Autodesk Fusion 360 part; units mm, degrees
sketch "Sketch1" plane through (0, 0, 0) normal (0, 0, 1) x (1, 0, 0)
  circle A0 centre (0, 0) radius 31.75
  circle A1 centre (0, 0) radius 25.4
  dimension "d1" = 63.5
  dimension "d2" = 50.8
extrude "Extrude1" add sketch "Sketch1" along normal blind 7.62 makes body 1
chamfer "Chamfer1" distance 3.175 distance2 3.175 1 edges at (-23.6811, 9.185, 7.62) measured on face at (29.4206, -2.8393, 7.62) on bodies 1
sketch "Sketch2" plane through (0, 0, 0) normal (1, 0, 0) x (0, 1, 0)
  arc A0 (-31.115, 59.4476) -> (-33.147, 7.7483) centre (-9.0465, 32.6906) ccw
  arc A1 (-46.5417, 59.4476) -> (-33.147, 0) centre (-13.9818, 35.5511) ccw
  line L0 (-33.147, 7.7483) -> (-33.147, 0)
  line L1 (-33.147, 7.7483) -> (-29.083, 7.7483)
  line L2 (-29.083, 7.7483) -> (-29.083, 0)
  line L3 (-29.083, 0) -> (-33.147, 0)
  line L4 (-33.147, 0) -> (-33.147, 7.7483)
  line L5 (-31.115, 0) -> (-31.115, 59.4476) construction
  line L6 (-46.5417, 59.4476) -> (-31.115, 59.4476)
extrude "Extrude2" add sketch "Sketch2" along normal blind 7.62 bodies 1
sketch "Sketch5" plane through (0, 0, 59.4476) normal (0, 0, 1) x (-1, 0, 0)
  line L0 (0, 31.115) -> (0, 46.5417)
  line L1 (0, 46.5417) -> (-7.62, 46.5417)
  line L2 (-7.62, 46.5417) -> (-7.62, 31.115)
  line L3 (-7.62, 31.115) -> (0, 31.115)
  line L4 (12.7, 39.2684) -> (-12.7, 39.2684) construction
  line L5 (-12.7, 39.2684) -> (-12.7, -39.2684) construction
  line L6 (-12.7, -39.2684) -> (12.7, -39.2684) construction
  line L7 (12.7, -39.2684) -> (12.7, 39.2684) construction
  line L8 (12.7, 39.2684) -> (-12.7, -39.2684) construction
  line L9 (-12.7, 39.2684) -> (12.7, -39.2684) construction
  arc A0 (12.7, -39.2684) -> (12.7, 39.2684) centre (-69.8788, 0) ccw
  arc A1 (12.7, 39.2684) -> (-12.7, 39.2684) centre (0, -0.0042) ccw
  arc A2 (-12.7, 39.2684) -> (-12.7, -39.2684) centre (69.8788, 0) ccw
  arc A3 (-12.7, -39.2684) -> (12.7, -39.2684) centre (0, 0.0042) ccw
  line L10 (0, 46.5417) -> (-7.62, 46.5417)
  line L11 (-7.62, 46.5417) -> (-7.62, 31.115)
  line L12 (-7.62, 31.115) -> (0, 31.115)
  line L13 (0, 31.115) -> (0, 46.5417)
  dimension "d20" = 25.4
  dimension "d21" = 78.5368
  dimension "d22" = 91.44
  dimension "d23" = 41.275
  dimension "d24" = 91.44
  dimension "d25" = 41.275
extrude "Extrude3" add sketch "Sketch5" along normal blind 5.08 separate body contours L0 L2 L3 A0 A1 A2 A3 L11 L12 L13 makes body 2
extrude "Extrude4" add 1 faces at (2.54, -36.2572, 59.4476) along direction (0, 0, 1) blind 5.08 on bodies 1 bodies 1 2
fillet "Fillet1" radius 6.35 1 edges at (12.7, 39.2684, 61.9876) on bodies 1
fillet "Fillet2" radius 6.35 1 edges at (-12.7, 39.2684, 61.9876) on bodies 1
sketch "Sketch6" plane through (0, 0, 64.5276) normal (0, 0, 1) x (-1, 0, 0)
  arc A0 (9.6213, -40.1338) -> (13.9635, -36.4929) centre (8.1411, -33.9587) ccw
  arc A1 (13.9635, -36.4929) -> (12.7, 39.2684) centre (-69.8788, 0) ccw
  arc A2 (12.7, 39.2684) -> (0, 41.2708) centre (0, -0.0042) ccw
  line L0 (0, 41.2708) -> (0, 46.5417)
  line L1 (0, 46.5417) -> (-7.62, 46.5417)
  line L2 (-7.62, 46.5417) -> (-7.62, 40.5613)
  arc A3 (-7.62, 40.5613) -> (-12.7, 39.2684) centre (0, -0.0042) ccw
  arc A4 (-12.7, 39.2684) -> (-13.9635, -36.4929) centre (69.8788, 0) ccw
  arc A5 (-13.9635, -36.4929) -> (-9.6213, -40.1338) centre (-8.1411, -33.9587) ccw
  arc A6 (-9.6213, -40.1338) -> (9.6213, -40.1338) centre (0, 0.0042) ccw
  circle A7 centre (-0.3341, 0.0042) radius 12.7
  dimension "d35" = 25.4
extrude "Extrude5" cut sketch "Sketch6" against normal blind 5.08 contours A7 bodies 1
chamfer "Chamfer2" distance 3.175 angle 45 1 edges at (12.1747, 4.5883, 59.4476) on bodies 1
sketch "Sketch7" plane through (0, 0, 64.5276) normal (0, 0, 1) x (-1, 0, 0)
  circle A0 centre (-0.3341, 0.0042) radius 12.7
  arc A1 (9.6213, -40.1338) -> (13.9635, -36.4929) centre (8.1411, -33.9587) ccw
  arc A2 (13.9635, -36.4929) -> (12.7, 39.2684) centre (-69.8788, 0) ccw
  arc A3 (12.7, 39.2684) -> (0, 41.2708) centre (0, -0.0042) ccw
  line L0 (0, 41.2708) -> (0, 46.5417)
  line L1 (0, 46.5417) -> (-7.62, 46.5417)
  line L2 (-7.62, 46.5417) -> (-7.62, 40.5613)
  arc A4 (-7.62, 40.5613) -> (-12.7, 39.2684) centre (0, -0.0042) ccw
  arc A5 (-12.7, 39.2684) -> (-13.9635, -36.4929) centre (69.8788, 0) ccw
  arc A6 (-13.9635, -36.4929) -> (-9.6213, -40.1338) centre (-8.1411, -33.9587) ccw
  arc A7 (-9.6213, -40.1338) -> (9.6213, -40.1338) centre (0, 0.0042) ccw
  line L3 (3.81, 25.4) -> (-3.81, 25.4)
  line L4 (-3.81, 25.4) -> (-3.81, -25.4)
  line L5 (-3.81, -25.4) -> (3.81, -25.4)
  line L6 (3.81, -25.4) -> (3.81, 25.4)
  line L7 (3.81, 25.4) -> (-3.81, -25.4) construction
  line L8 (-3.81, 25.4) -> (3.81, -25.4) construction
  dimension "d39" = 7.62
  dimension "d40" = 50.8
extrude "Extrude6" add sketch "Sketch7" along normal blind 12.7 contours A0 L4 L6 | A0 L3 L4 L6 | A0 L4 L5 L6 bodies 1
fillet "Fillet3" radius 6.35 1 edges at (0, -25.4, 64.5276) on bodies 1
fillet "Fillet4" radius 6.35 1 edges at (0, 25.4, 64.5276) on bodies 1
sketch "Sketch10" plane through (0, 0, 0) normal (1, 0, 0) x (0, 1, 0)
  line L0 (-31.75, 0) -> (-42.7767, -62.5353)
  line L1 (-31.75, 0) -> (31.75, 0) construction
  line L2 (-31.75, 0) -> (-25.4, 0)
  line L3 (-25.4, 0) -> (-36.4267, -62.5353)
  line L4 (-25.4, 0) -> (38.1, 0) construction
  line L5 (-36.4267, -62.5353) -> (-49.1267, -62.5353)
  line L6 (-49.1267, -62.5353) -> (-49.1267, -67.6153)
  line L7 (-49.1267, -67.6153) -> (-36.4267, -67.6153)
  line L8 (-36.4267, -67.6153) -> (-36.4267, -62.5353)
  dimension "d57" = 100
  dimension "d58" = 63.5
  dimension "d59" = 6.35
  dimension "d60" = 100
  dimension "d61" = 63.5
  dimension "d62" = 12.7
  dimension "d63" = 5.08
revolve "Revolve2" add sketch "Sketch10" angle 10 about axis through (0, 0, 1.75) along (0, 0, 1) bodies 1
pattern_circular "C-Pattern1" count 3 over 360 about axis through (0, 0, 1.75) along (0, 0, 1) of "Revolve2"
sketch "Sketch11" plane through (0, 0, 7.62) normal (0, 0, 1) x (-1, 0, 0)
  circle A0 centre (0, 0) radius 28.575
  line L0 (0, 31.75) -> (0, 29.083)
  line L1 (0, 29.083) -> (-7.62, 29.083)
  line L2 (-7.62, 29.083) -> (-7.62, 30.822)
  arc A1 (-7.62, 30.822) -> (0, 31.75) centre (0, 0) ccw
  line L3 (-27.4963, -15.875) -> (-37.0457, -21.3883)
  arc A2 (-37.0457, -21.3883) -> (-32.7688, -27.4963) centre (0, 0) ccw
  line L4 (-32.7688, -27.4963) -> (-24.3219, -20.4085)
  arc A3 (-27.4963, -15.875) -> (-24.3219, -20.4085) centre (0, 0) ccw
  line L5 (27.4963, -15.875) -> (37.0457, -21.3883)
  arc A4 (37.0457, -21.3883) -> (40.1969, -14.6305) centre (0, 0) ccw
  line L6 (40.1969, -14.6305) -> (29.8352, -10.8591)
  arc A5 (27.4963, -15.875) -> (29.8352, -10.8591) centre (0, 0) ccw
  line L7 (27.4963, -15.875) -> (10.16, -5.9004)
  line L8 (-24.3219, -20.4085) -> (-11.3582, -5.9004)
  line L9 (-11.3582, -5.9004) -> (10.16, -5.9004)
  line L10 (-32.7688, -27.4963) -> (0, -40.64)
  line L11 (0, -40.64) -> (37.0457, -21.3883)
extrude "Extrude7" cut sketch "Sketch11" against normal blind 17.78 contours A0 L7 L8 L9 | A0 A1 L7 L8 | A1 L4 L5 L10 L11 picked at (-0.3547, -13.4585) bodies 1
The listing builds one solid part. Answer for the finished solid, in the listing's coordinates (mm). A direction names the side the tool comes from. Round coordinates to 2 decimals unless told otherwise and drop trailing zeros. Loops run counter-clockwise (first coordinate to the right, second up) from the corner with the lowest first, then second, coordinate; pieces in that order, holes last.
Q1. Section A-A, the plane z = -50.5 is taken. Determine the outline of the cut face in (x, y), then the cut area to 3 significant figures.
Q2. Section B-B, the plane y = 2 is taken. Count the separate pieces of the cut face and the enclosed holes in it, then the cut area to 3 significant figures.
Q3. Section C-C, the plane y = 34 is taken. Determine the outline of the cut face in (x, z).
Q4. For a pull along Y with two mould halves and no side action, classify faces 5 (the face through (-38, 18, -67.615)), 6 (the face through (-0.05, 27.31, 66.34)), 7 (the face through (-5.53, 11.26, 63.59)) as released by +Y, released by -Y, zero draft, split by the parting line, or undercut.
Q5. Given pin 1 Ø5.5 at (x, y) = (2.5, -47) entering from +Z; pin 2 Ø3 at (x, y) = (38, 29) entering from +Z; pin 3 Ø1.9 at (x, z) = (-1, 75) entering from -Y; pin 4 Ø10 at (x, z) = (-11, -8.5) entering from +Y, each flat-ended and moving along its own axis, determine where each tip first touches the part or whether it passes through.
Q6. Which of the six approach directions +Z, -Z, +X, -X, +Y, -Y give full straight-line access (tool end or side, diameter ignored) to faces 1 (the face through (0, 0, 64.528)), 2 (the face through (4, -31, 7.748)), 3 (the face through (-42, 19, -62.535)), 4 (the face through (0, 25.4, 74))?
Q7. Find the intervals of material crossed by line 1 (X direction, y = 0, z = 1.75); line 2 (Z direction, x = 29, y = -8.5); line 3 (X direction, y = -17.5, z = 71.5), in increasing order.
Completed:
1. outline: (-38.2, 13.9) - (-32.24, 11.73) arc R34.3 cw to (-29.71, 17.15) - (-35.21, 20.33) arc R40.65 ccw to start; (0, -40.65) arc R40.65 ccw to (7.06, -40.04) - (5.96, -33.78) arc R34.3 cw to (0, -34.3) - close; (26.28, 22.05) arc R34.3 cw to (29.71, 17.15) - (35.21, 20.33) arc R40.65 ccw to (31.14, 26.13) - close
1. area: 125 mm2
2. separate pieces: 5
2. enclosed holes: 0
2. area: 265 mm2
3. outline: (-15.01, 59.45) - (15.01, 59.45) - (15.01, 64.53) - (-15.01, 64.53) - close
4. face 5: zero draft
4. face 6: released by +Y
4. face 7: undercut
5. pin 1: stops at z = 64.53
5. pin 2: stops at z = -62.54
5. pin 3: stops at y = -25.4
5. pin 4: passes through
6. face 1: -Z
6. face 2: +X, -X, +Y
6. face 3: +Z, -X, +Y
6. face 4: +Z, +X, -X, +Y
7. line 1: x = -31.75 to -25.4, 25.4 to 31.75
7. line 2: z = 0 to 7.62
7. line 3: x = -3.81 to 3.81
